Read the model definition and answer for the solid it produces. Units are mm, in the model's axes. Face numbers are marked on the shaded views. A direction names the side the tool comes from. Give positions to 0.01 mm unless a question says otherwise; leave off trailing zeros. Order: outer loops, then holes, each group sorted by start corner. A loop starts at its lowest first (then second) coordinate and runs counter-clockwise, first axis right, second up. Notation, with made-up numbers: (30.25, 32) - (84.25, 32) arc R19 cw to (84.25, 64) - close; hole circle Ø10 at (62.5, 7). An arc over 180 degrees is marked (long way). Use a Markdown table: item, result. Add a question column.
1. A cutting plane is placed at B-B on x = 11.5. Determine the outline of the cut face in (y, z), and give its area (3 significant figures).
2. Which of the six approach directions +Z, -Z, +X, -X, +Y, -Y give full straight-line access (tool end or side, diameter ignored) to the marked faces 1 and 2?
3. Flat-ended cylindrical pins translate along their axes: P1, Ø0.9, axis at x = 1, y = 0, coming from the +Z side; P2, Ø1.5, axis at x = 2, y = 1.5, coming from the -Z side; P3, Ø2, axis at y = 0, z = 2, coming from the -X side; P4, Ø1, axis at x = 5.5, y = -0.5, coming from the -Z side. Find the tip coordinate at first contact, or state that the pin passes through.
4. For a pull along Z with two mould halves and no side action, classify the marked faces 3, 4, 5 and 6 as released by +Z, released by -Z, zero draft, split by the parting line, or undercut.
5. A cutting plane is placed at A-A on y = 0. Determine the outline of the cut face in (x, z).
6. Consider L1, parallel to X at y = 0.3, z = 0; L2, parallel to Y at x = 7.5, z = 0.1; L3, parallel to Z at x = 4.5, y = -0.7. Determine where each line is inside the solid, lowest interval first.
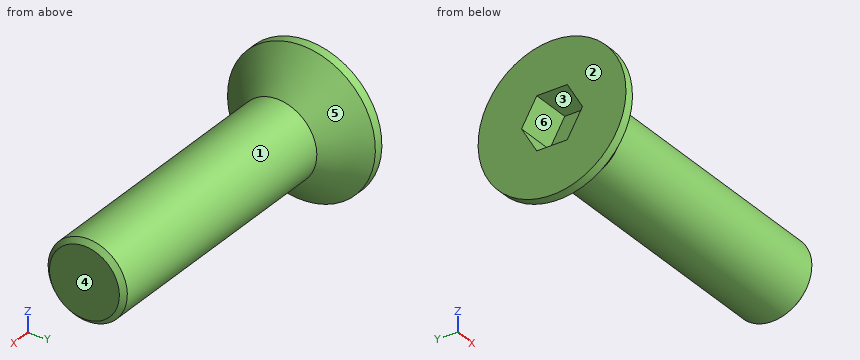
```python
from build123d import *

# Parameters (mm, degrees)
F3_DEPTH = 1.5


with BuildPart() as f1:
    # F0 (on Front) → F1 (revolve)
    with BuildSketch(Plane.XZ):
        Polygon((0, 2.8), (0, 0), (12, 0), (12, 1.323223), (11.823223, 1.5), (1.65, 1.5), (0.35, 2.8), align=None)
    revolve(axis=Axis((6, 0, 0), (1, 0, 0)))

    # F2 (on face) → F3 (cut)
    with BuildSketch(Plane(origin=(0, 0, 0), x_dir=(0, -1, 0), z_dir=(-1, 0, 0))):
        Polygon((1.154701, 0), (0.57735, 1), (-0.57735, 1), (-1.154701, 0), (-0.57735, -1), (0.57735, -1), align=None)
    extrude(amount=-F3_DEPTH, mode=Mode.SUBTRACT)


solid = f1.part
```
Output values:
| question | item | result |
|---|---|---|
| 1 | outline | circle Ø3 at (0, 0) |
| 1 | area | 7.07 mm² |
| 2 | face 1 | +X |
| 2 | face 2 | +Z, -Z, -X, +Y, -Y |
| 3 | P1 | z = 2.6 |
| 3 | P2 | z = -1.41 |
| 3 | P3 | x = 0 |
| 3 | P4 | z = -1.5 |
| 4 | face 3 | undercut |
| 4 | face 4 | zero draft |
| 4 | face 5 | split by the parting line |
| 4 | face 6 | undercut |
| 5 | outline | (0, -2.8) - (0.35, -2.8) - (1.65, -1.5) - (11.82, -1.5) - (12, -1.32) - (12, 1.32) - (11.82, 1.5) - (1.65, 1.5) - (0.35, 2.8) - (0, 2.8) - (0, 1) - (1.5, 1) - (1.5, -1) - (0, -1) - close |
| 6 | L1 | 1.5 to 12 |
| 6 | L2 | -1.5 to 1.5 |
| 6 | L3 | -1.33 to 1.33 |
